Verification items for the finished model (mm, model axes). Face numbers are marked on the shaded views. A direction names the side the tool comes from. Give positions to 0.01 mm unless a question says otherwise; leave off trailing zeros. Order: outer loops, then holes, each group sorted by start corner. A loop starts at its lowest first (then second) coordinate and runs counter-clockwise, first axis right, second up.
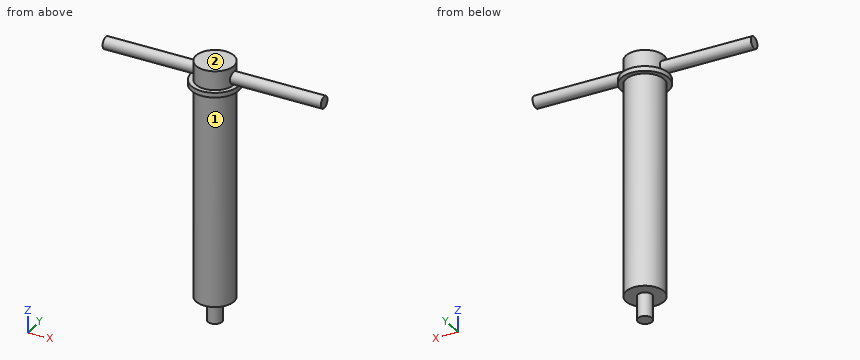
from build123d import *

# Parameters (mm, degrees)
SKETCH1_R           = 4
BOSS_EXTRUDE1_DEPTH = 50
SKETCH2_R           = 5
BOSS_EXTRUDE2_DEPTH = 1
SKETCH3_R           = 1.25
BOSS_EXTRUDE3_DEPTH = 23
SKETCH4_R           = 1.5
BOSS_EXTRUDE4_DEPTH = 5


with BuildPart() as part:
    # Sketch1 → Boss-Extrude1 (new body)
    with BuildSketch(Plane.XY):
        Circle(SKETCH1_R)
    extrude(amount=BOSS_EXTRUDE1_DEPTH)

    # Sketch2 → Boss-Extrude2 (add)
    with BuildSketch(Plane.XY.offset(46)):
        Circle(SKETCH2_R)
    extrude(amount=-BOSS_EXTRUDE2_DEPTH)

    # Sketch3 → Boss-Extrude3 (add, symmetric)
    with BuildSketch(Plane(origin=(0, 0, 0), x_dir=(0, 0, -1), z_dir=(1, 0, 0))):
        with Locations((-47.5, 0)):
            Circle(SKETCH3_R)
    extrude(amount=BOSS_EXTRUDE3_DEPTH, both=True)

    # Sketch4 → Boss-Extrude4 (add)
    with BuildSketch(Plane(origin=(0, 0, 0), x_dir=(-1, 0, 0), z_dir=(0, 0, -1))):
        Circle(SKETCH4_R)
    extrude(amount=BOSS_EXTRUDE4_DEPTH)


solid = part.part
(1) Scan lines: line 1 (Z direction, x = 2.5, y = -3.5); line 2 (Z direction, x = 4.5, y = 0.75); line 3 (X direction, y = -2.75, z = 33). Record each from-to range of solid material in increasing order.
Solved:
line 1: z = 45 to 46
line 2: z = 45 to 46, 46.5 to 48.5
line 3: x = -2.9 to 2.9
(2) Section check D-D, the plane z = 27.5. Enter the section's corners in (x, y).
Solved:
outline: circle Ø8 at (0, 0)
(3) Section check A-A, the plane y = 0. Enter the section's corners in (x, z).
Solved:
outline: (-23, 46.25) - (-4, 46.25) - (-4, 46) - (-5, 46) - (-5, 45) - (-4, 45) - (-4, 0) - (-1.5, 0) - (-1.5, -5) - (1.5, -5) - (1.5, 0) - (4, 0) - (4, 45) - (5, 45) - (5, 46) - (4, 46) - (4, 46.25) - (23, 46.25) - (23, 48.75) - (4, 48.75) - (4, 50) - (-4, 50) - (-4, 48.75) - (-23, 48.75) - close
(4) Set-up check for the marked faces 1 and 2: record each of +Z, -Z, +X, -X, +Y, -Y from which the full face is reachable in a straight line by a thin tool's end or side.
Solved:
face 1: -Z
face 2: +Z, +X, -X, +Y, -Y
(5) Section check C-C, the plane x = 10. Enter the section's corners in (y, z).
Solved:
outline: circle Ø2.5 at (0, 47.5)
(6) Section check B-B, the plane z = 47.5. Enter the section's corners in (x, y).
Solved:
outline: (-23, -1.25) - (-3.8, -1.25) arc R4 ccw to (3.8, -1.25) - (23, -1.25) - (23, 1.25) - (3.8, 1.25) arc R4 ccw to (-3.8, 1.25) - (-23, 1.25) - close
(7) Go/stop test with flat-tipped pins: pin 1 (4 mm diameter, centred on x = -16, y = 1, fed in from +Z); pin 2 (1 mm diameter, centred on x = 2.5, z = 10.5, fed in from -Y); pin 3 (2 mm diameter, centred on y = -1, z = 6, fed in from +X). Record where each tip stops, or that it passes through.
Solved:
pin 1: stops at z = 48.75
pin 2: stops at y = -3.46
pin 3: stops at x = 4
